```python
from build123d import *

# Parameters (mm, degrees)
SKETCH1_W               = 254
SKETCH1_H               = 254
PLATFORM_BASE_DEPTH     = 7.62
CORNER_ROUNDING_R       = 25.4
SKETCH3_R               = 1.75
CUT_EXTRUDE1_DEPTH      = 180.766694357
SKETCH4_W               = 63.5
SKETCH4_H               = 30.48
CUT_EXTRUDE2_DEPTH      = 180.766694357
SKETCH6_W               = 12.7
SKETCH6_H               = 7.62
CUT_EXTRUDE3_DEPTH      = 180.766694357
MIRROR5_COPY_1_SKETCH_W = 12.7
MIRROR5_COPY_1_SKETCH_H = 7.62
MIRROR5_COPY_1_DEPTH    = 180.766694357
SKETCH8_W               = 7.62
SKETCH8_H               = 12.7
CUT_EXTRUDE4_DEPTH      = 180.766694357
MIRROR7_COPY_1_SKETCH_W = 7.62
MIRROR7_COPY_1_SKETCH_H = 12.7
MIRROR7_COPY_1_DEPTH    = 180.766694357


with BuildPart() as part:
    # Sketch1 → Platform-Base (new body)
    with BuildSketch(Plane(origin=(0, 0, 0), x_dir=(1, 0, 0), z_dir=(0, 1, 0))):
        Rectangle(SKETCH1_W, SKETCH1_H)
    extrude(amount=PLATFORM_BASE_DEPTH)

    # Corner-Rounding
    corner_rounding_edges = [part.edges().sort_by_distance(p)[0] for p in [
        (127, 3.81, 127),
        (-127, 3.81, 127),
        (-127, 3.81, -127),
        (127, 3.81, -127),
    ]]
    fillet(corner_rounding_edges, radius=CORNER_ROUNDING_R)

    # Sketch3 → Cut-Extrude1 (cut, through all)
    with BuildSketch(Plane(origin=(0, 7.62, 0), x_dir=(1, 0, 0), z_dir=(0, 1, 0))):
        with Locations(Location((15, -38.8, 0), (0, 0, 270))):
            Circle(SKETCH3_R)
        with Locations(Location((15, -62.8, 0), (0, 0, 270))):
            Circle(SKETCH3_R)
        with Locations(Location((-15, -62.8, 0), (0, 0, 270))):
            Circle(SKETCH3_R)
        with Locations(Location((-15, -38.8, 0), (0, 0, 270))):
            Circle(SKETCH3_R)
    cut_extrude1 = extrude(amount=-CUT_EXTRUDE1_DEPTH, mode=Mode.SUBTRACT)

    # Mirror2: Cut-Extrude1 across plane
    add(cut_extrude1.mirror(Plane.XY), mode=Mode.SUBTRACT)

    # Sketch4 → Cut-Extrude2 (cut, through all)
    with BuildSketch(Plane(origin=(0, 7.62, 0), x_dir=(1, 0, 0), z_dir=(0, 1, 0))):
        with Locations((0, -87.63)):
            Rectangle(SKETCH4_W, SKETCH4_H)
    cut_extrude2 = extrude(amount=-CUT_EXTRUDE2_DEPTH, mode=Mode.SUBTRACT)

    # Mirror3: Cut-Extrude2 across plane
    add(cut_extrude2.mirror(Plane.XY), mode=Mode.SUBTRACT)

    # Sketch6 → Cut-Extrude3 (cut, through all)
    with BuildSketch(Plane(origin=(0, 7.62, 0), x_dir=(1, 0, 0), z_dir=(0, 1, 0))):
        with Locations((-76.2, -123.19)):
            Rectangle(SKETCH6_W, SKETCH6_H)
    cut_extrude3 = extrude(amount=-CUT_EXTRUDE3_DEPTH, mode=Mode.SUBTRACT)

    # Mirror4: Cut-Extrude3 across plane
    add(cut_extrude3.mirror(Plane.XY), mode=Mode.SUBTRACT)

    # Mirror5: Cut-Extrude3 across plane
    add(cut_extrude3.mirror(Plane.ZY), mode=Mode.SUBTRACT)

    # Mirror5 copy 1 sketch → Mirror5 copy 1 (cut, through all)
    with BuildSketch(Plane(origin=(0, 7.62, 0), x_dir=(-1, 0, 0), z_dir=(0, 1, 0))):
        with Locations((-76.2, -123.19)):
            Rectangle(MIRROR5_COPY_1_SKETCH_W, MIRROR5_COPY_1_SKETCH_H)
    extrude(amount=-MIRROR5_COPY_1_DEPTH, mode=Mode.SUBTRACT)

    # Sketch8 → Cut-Extrude4 (cut, through all)
    with BuildSketch(Plane(origin=(0, 7.62, 0), x_dir=(1, 0, 0), z_dir=(0, 1, 0))):
        with Locations((-123.19, -76.2)):
            Rectangle(SKETCH8_W, SKETCH8_H)
    cut_extrude4 = extrude(amount=-CUT_EXTRUDE4_DEPTH, mode=Mode.SUBTRACT)

    # Mirror6: Cut-Extrude4 across plane
    add(cut_extrude4.mirror(Plane.XY), mode=Mode.SUBTRACT)

    # Mirror7: Cut-Extrude4 across plane
    add(cut_extrude4.mirror(Plane.ZY), mode=Mode.SUBTRACT)

    # Mirror7 copy 1 sketch → Mirror7 copy 1 (cut, through all)
    with BuildSketch(Plane(origin=(0, 7.62, 0), x_dir=(-1, 0, 0), z_dir=(0, 1, 0))):
        with Locations((-123.19, -76.2)):
            Rectangle(MIRROR7_COPY_1_SKETCH_W, MIRROR7_COPY_1_SKETCH_H)
    extrude(amount=-MIRROR7_COPY_1_DEPTH, mode=Mode.SUBTRACT)


solid = part.part
```
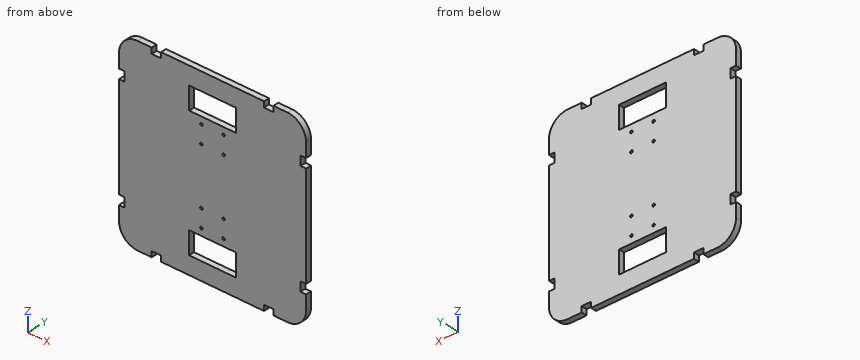
Input: part model. Units: mm. Frame: model coordinates. Give positions to 0.01 mm unless a question says otherwise; leave off trailing zeros. Loops run counter-clockwise (first coordinate to the right, second up) from the corner with the lowest first, then second, coordinate; pieces in that order, holes last. Notation, with made-up numbers: M -33,-22.5 L -14,-22.5 A34 ccw -14,9.5 Z; hole C 36,-12.5 d6. An arc over 180 degrees is marked long. Answer as CSV lines item,"result". Start each with the question number.
1. Line query: L1, parallel to Z at x = -2, y = 7; L2, parallel to X at y = 1.75, z = 62.8; L3, parallel to X at y = 1.25, z = -89. Output: solid intervals per line, ascending.
2. Section B-B on y = 3. State how many separate pieces and enclosed holes the cut face has, plus the area to 3 significant figures.
3. Pin query (flat end, axial travel): P1, Ø4, axis at y = 5.5, z = 123, coming from the +X side; P2, Ø4, axis at x = -122, y = 3.5, coming from the +Z side; P3, Ø1, axis at y = 1.5, z = 79.5, coming from the -X side; P4, Ø3, axis at x = -15, z = -38.8, coming from the -Y side. Return the tip coordinate at first contact, or that it passes through.
4. Section A-A on z = -88. Return loops of the section in (x, y).
Computed values:
1,L1,"z = -127 to -102.87, -72.39 to 72.39, 102.87 to 127"
1,L2,"x = -127 to -16.75, -13.25 to 13.25, 16.75 to 127"
1,L3,"x = -127 to -31.75, 31.75 to 127"
2,separate pieces,"1"
2,enclosed holes,"10"
2,area,"59,200 mm²"
3,P1,"stops at x = 118"
3,P2,"stops at z = 119.11"
3,P3,"stops at x = -119.38"
3,P4,"passes through"
4,outline,"M -127,0 L -31.75,0 L -31.75,7.62 L -127,7.62 Z; M 31.75,0 L 127,0 L 127,7.62 L 31.75,7.62 Z"
